The model under review builds one solid part; all positions refer to its coordinate system, in mm. Coordinates: 2 decimals unless noted, no trailing zeros. Order: outer loops, then holes, each group sorted by start corner. A loop starts at its lowest first (then second) coordinate and runs counter-clockwise, first axis right, second up. Notation, with made-up numbers: M -5,32.25 L 50,32.25 A29 cw 50,55.25 Z; hole C 66.5,23.25 d6. An arc over 180 degrees is marked long. Answer as CSV lines item,"result". Start each with the question number.
Q1. Wall thickness on L1, parallel to X at y = 152.5, z = 8.25; L2, parallel to X at y = 83, z = 6.5; L3, parallel to Y at x = 155.5, z = 18.25: over which ranges is each line inside the solid? List them lowest first. Write a range as [from, to].
Q2. Consider section D-D on y = 209. Write out the cut boundary in (x, z).
Q3. For P1, Ø12, axis at y = 235, z = 11.5, coming from the +X side; P2, Ø12.5, axis at x = -452, z = 11, coming from the -Y side; P3, Ø1, axis at y = 147.5, z = 15, coming from the -X side, all flat-tipped, find the tip position at first contact; note any pin that passes through.
Q4. Consider section B-B on z = 19.25. Write out the cut boundary in (x, y), and give its area (3 significant figures).
Q5. Consider section C-C on x = 439.5. Write out the cut boundary in (y, z), and give its area (3 significant figures).
Q6. Consider section A-A on y = 141. Write out the cut boundary in (x, z).
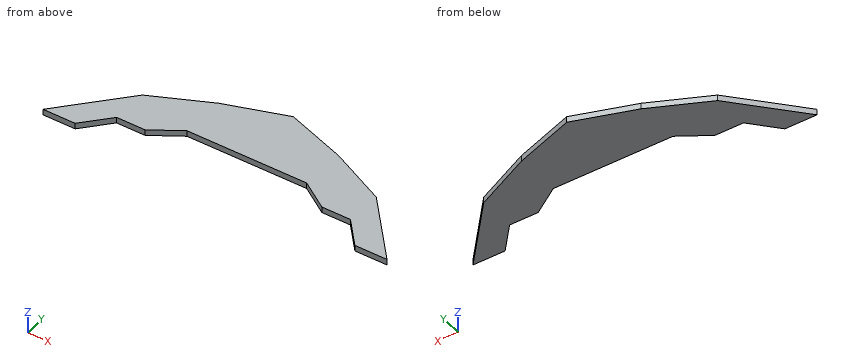
from build123d import *

# Parameters (mm, degrees)
F1_DEPTH = 25
F3_DEPTH = 25
F4_W     = 200
F4_H     = 100
F5_DEPTH = 25


with BuildPart() as f1:
    # F0 (on Top) → F1 (new body)
    with BuildSketch(Plane.XY):
        Polygon((-510, 271.8948125839), (-750, 0), (0, 0), (0, 271.8948125839), align=None)
        Polygon((-261, 390.4831971128), (-510, 271.8948125839), (0, 271.8948125839), (0, 390.4831971128), align=None)
        Polygon((0, 480.4831971128), (-261, 390.4831971128), (0, 390.4831971128), align=None)
        Polygon((0, 480.4831971128), (0, 390.4831971128), (261, 390.4831971128), align=None)
        Polygon((0, 390.4831971128), (0, 271.8948125839), (510, 271.8948125839), (261, 390.4831971128), align=None)
        Polygon((0, 271.8948125839), (0, 0), (750, 0), (510, 271.8948125839), align=None)
    extrude(amount=F1_DEPTH)

    # F2 (on face) → F3 (cut)
    with BuildSketch(Plane(origin=(0, 0, 0), x_dir=(1, 0, 0), z_dir=(0, 0, -1))):
        Polygon((610, 0), (-610, 0), (-510, -113.2895052433), (-385.5, -113.2895052433), (-261, -195.2415985564), (261, -195.2415985564), (385.5, -113.2895052433), (510, -113.2895052433), align=None)
    extrude(amount=-F3_DEPTH, mode=Mode.SUBTRACT)


with BuildPart() as f5:
    # F4 (on face) → F5 (new body)
    with BuildSketch(Plane.XY.offset(25)):
        with Locations((0, 145.2415985564)):
            Rectangle(F4_W, F4_H)
    extrude(amount=-F5_DEPTH)


solid = f1.part
Evaluation:
1,L1,"x = [-615.39, -325.93], [325.93, 615.39]"
1,L2,"x = [-676.74, -536.74], [536.74, 676.74]"
1,L3,"y = [195.24, 426.86]"
2,outline,"M -565.52,0 L 565.52,0 L 565.52,25 L -565.52,25 Z"
3,P1,"stops at x = 547.86"
3,P2,"stops at y = 113.29"
3,P3,"stops at x = -620.24"
4,outline,"M -750,0 L -610,0 L -510,113.29 L -385.5,113.29 L -261,195.24 L 261,195.24 L 385.5,113.29 L 510,113.29 L 610,0 L 750,0 L 510,271.89 L 261,390.48 L 0,480.48 L -261,390.48 L -510,271.89 Z"
4,area,"278,000 mm²"
5,outline,"M 113.29,0 L 305.47,0 L 305.47,25 L 113.29,25 Z"
5,area,"4,800 mm²"
6,outline,"M -625.54,0 L -343.4,0 L -343.4,25 L -625.54,25 Z; M 343.4,0 L 625.54,0 L 625.54,25 L 343.4,25 Z"
